CAD build for the part. Positions are in the model's coordinates, mm. A direction names the side the tool comes from. Give positions to 0.01 mm unless a question says otherwise; leave off trailing zeros. Loops run counter-clockwise (first coordinate to the right, second up) from the corner with the lowest first, then second, coordinate; pieces in that order, holes last.
Autodesk Inventor part; units mm, degrees
ref_plane "YZ Plane" through (0, 0, 0) normal (1, 0, 0) x (0, 1, 0)
ref_plane "XZ Plane" through (0, 0, 0) normal (0, 1, 0) x (-1, 0, 0)
ref_plane "XY Plane" through (0, 0, 0) normal (0, 0, 1) x (1, 0, 0)
sketch "草圖17" plane through (0, 0, 0) normal (0, 0, 1) x (1, 0, 0)
  line L0 (-12.5, -3) -> (12.5, -3)
  line L1 (12.5, -3) -> (12.5, 3)
  line L2 (12.5, 3) -> (-12.5, 3)
  line L3 (-12.5, 3) -> (-12.5, -3)
  line L4 (-12.5, -3) -> (12.5, 3) construction
  line L5 (12.5, -3) -> (-12.5, 3) construction
  line L6 (0, 0) -> (-6.6625, 0) construction
  circle A0 centre (9.5, 0) radius 2
  line L7 (-2.5, 0) -> (-4.5, 0) construction
  line L8 (-2.5, 1) -> (-4.5, 1)
  line L9 (-4.5, -1) -> (-2.5, -1)
  arc A1 (-2.5, -1) -> (-2.5, 1) centre (-2.5, 0) ccw
  arc A2 (-4.5, 1) -> (-4.5, -1) centre (-4.5, 0) ccw
  line L10 (5.5, -0.0384) -> (3.5, -0.0384) construction
  line L11 (5.5, 0.9616) -> (3.5, 0.9616)
  line L12 (3.5, -1.0384) -> (5.5, -1.0384)
  arc A3 (5.5, -1.0384) -> (5.5, 0.9616) centre (5.5, -0.0384) ccw
  arc A4 (3.5, 0.9616) -> (3.5, -1.0384) centre (3.5, -0.0384) ccw
  line L13 (7.5, 3) -> (7.5, -3)
  point P0 (-3.5, 0)
  point P1 (4.5, -0.0384)
  dimension "d166" = 25
  dimension "d167" = 6
  dimension "d170" = 4
  dimension "d171" = 3
  dimension "d173" = 2
  dimension "d174" = 12
  dimension "d175" = 2
  dimension "d190" = 4
  dimension "d191" = 2
  dimension "d192" = 2
extrude "擠出18" add sketch "草圖17" along normal mid plane 4 contours L3 L2 L13 L0
sketch "草圖18" plane through (0, 0, 0) normal (0, 0, 1) x (1, 0, 0)
  line L0 (7.5, -3) -> (-12.5, -3)
  line L1 (-12.5, -3) -> (-12.5, 3)
  line L2 (-12.5, 3) -> (7.5, 3)
  arc A0 (-2.5, -1) -> (-2.5, 1) centre (-2.5, 0) ccw
  line L3 (-2.5, 1) -> (-4.5, 1)
  arc A1 (-4.5, 1) -> (-4.5, -1) centre (-4.5, 0) ccw
  line L4 (-4.5, -1) -> (-2.5, -1)
  line L5 (-12.5, -5.1) -> (-21.5, -5.1)
  line L6 (-21.5, -5.1) -> (-21.5, 5.1)
  line L7 (-21.5, 5.1) -> (-12.5, 5.1)
  line L8 (-12.5, 5.1) -> (-12.5, -5.1)
  line L9 (-12.5, -5.1) -> (-21.5, 5.1) construction
  line L10 (-21.5, -5.1) -> (-12.5, 5.1) construction
  arc A2 (-2.5, -1) -> (-2.5, 1) centre (-2.5, 0) ccw construction
  line L11 (-2.5, 0) -> (-4.5, 0) construction
  line L12 (-21.5, 0) -> (-31.5, 0) construction
  line L13 (-21.5, 2.1) -> (-31.5, 2.1)
  line L14 (-31.5, -2.1) -> (-21.5, -2.1)
  arc A3 (-21.5, -2.1) -> (-21.5, 2.1) centre (-21.5, 0) ccw
  arc A4 (-31.5, 2.1) -> (-31.5, -2.1) centre (-31.5, 0) ccw
  line L15 (-31.5, 5.1) -> (-21.5, 5.1)
  arc A5 (-21.5, -5.1) -> (-21.5, 5.1) centre (-21.5, 0) ccw
  line L16 (-21.5, -5.1) -> (-31.5, -5.1)
  arc A6 (-31.5, 5.1) -> (-31.5, -5.1) centre (-31.5, 0) ccw
  line L17 (-12.5, -3) -> (-12.5, 3) construction
  line L18 (7.5, 3) -> (7.5, -3)
  point P0 (0, 0)
  point P1 (-17, 0)
  point P2 (-26.5, 0)
  dimension "d181" = 2.1
  dimension "d182" = 10
  dimension "d183" = 3
  dimension "d189" = 9
extrude "擠出19" add sketch "草圖18" along normal mid plane 11 contours L8 L5 A5 L7 L1 | L16 A6 L15 L6 L13 A4 L14 | L6 A3 A5
sketch "草圖19" plane through (0, 0, 0) normal (0, 0, 1) x (1, 0, 0)
  arc A0 (-31.5, 5.1) -> (-31.5, -5.1) centre (-31.5, 0) ccw
  line L0 (-31.5, 5.1) -> (-12.5, 5.1)
  line L1 (-12.5, 5.1) -> (-12.5, -5.1)
  line L2 (-12.5, -5.1) -> (-31.5, -5.1)
  arc A1 (-21.5, -2.1) -> (-21.5, 2.1) centre (-21.5, 0) ccw
  line L3 (-21.5, 2.1) -> (-31.5, 2.1)
  arc A2 (-31.5, 2.1) -> (-31.5, -2.1) centre (-31.5, 0) ccw
  line L4 (-31.5, -2.1) -> (-21.5, -2.1)
  line L5 (-15.5, -5.1) -> (-45.605, -5.1)
  line L6 (-45.605, -5.1) -> (-45.605, 5.1)
  line L7 (-45.605, 5.1) -> (-15.5, 5.1)
  line L8 (-15.5, 5.1) -> (-15.5, -5.1)
  line L9 (-31.5, 5.1) -> (-12.5, 5.1)
  point P0 (0, 0)
  point P1 (-15.5, 5.1)
  dimension "d186" = 3
extrude "擠出20" cut sketch "草圖19" along normal mid plane 7 contours L0 L8 L2 A0 | A0 L5 L6 L7
sketch "草圖20" plane through (7.5, 3, 2) normal (0, 1, 0) x (1, 0, 0)
  line L0 (0, 0) -> (-20, 0)
  line L1 (-20, 0) -> (0, 0)
  line L2 (0, 4) -> (0, 0)
  point P0 (-7.5, 2)
  dimension "d193" = 20
  dimension "d194" = 0
extrude "擠出21" [suppressed]
properties part number "fan_holder_0301"
1. Saw through at B-B, the plane x = -17. List the corners of the cut face in (y, z).
Responses:
outline: (-5.1, -5.5) - (5.1, -5.5) - (5.1, -3.5) - (-5.1, -3.5) - close; (-5.1, 3.5) - (5.1, 3.5) - (5.1, 5.5) - (-5.1, 5.5) - close
2. Saw through at C-C, the plane x = -27. List the corners of the cut face in (y, z).
Responses:
outline: (-5.1, -5.5) - (-2.1, -5.5) - (-2.1, -3.5) - (-5.1, -3.5) - close; (-5.1, 3.5) - (-2.1, 3.5) - (-2.1, 5.5) - (-5.1, 5.5) - close; (2.1, -5.5) - (5.1, -5.5) - (5.1, -3.5) - (2.1, -3.5) - close; (2.1, 3.5) - (5.1, 3.5) - (5.1, 5.5) - (2.1, 5.5) - close
3. Tool access for faces 1 (the face through (-2.6, 1.4, -2)), 2 (the face through (-3, -3, 0)), 3 (the face through (2.5, -0.1, 0)), 4 (the face through (-26.2, 2.3, -3.5)): list every direction of +Z, -Z, +X, -X, +Y, -Y with a clear straight run to the whole face (end or side of a thin tool).
Responses:
face 1: -Z, +X, +Y, -Y
face 2: +Z, -Z, +X, -Y
face 3: +Z, -Z
face 4: -X, +Y, -Y
4. Saw through at A-A, the plane z = 1.5. List the corners of the cut face in (x, y).
Responses:
outline: (-15.5, -5.1) - (-12.5, -5.1) - (-12.5, -3) - (7.5, -3) - (7.5, 3) - (-12.5, 3) - (-12.5, 5.1) - (-15.5, 5.1) - close; hole (-4.5, -1) - (-2.5, -1) arc R1 ccw to (-2.5, 1) - (-4.5, 1) arc R1 ccw to start; hole (3.5, -1.04) - (5.5, -1.04) arc R1 ccw to (5.5, 0.96) - (3.5, 0.96) arc R1 ccw to start
5. Saw through at D-D, the plane z = 4.5. List the corners of the cut face in (x, y), and give its area (3 significant figures).
Responses:
outline: (-31.5, -5.1) - (-12.5, -5.1) - (-12.5, 5.1) - (-31.5, 5.1) arc R5.1 ccw to start; hole (-31.5, -2.1) - (-21.5, -2.1) arc R2.1 ccw to (-21.5, 2.1) - (-31.5, 2.1) arc R2.1 ccw to start
area: 179 mm2
6. Probe line 1 along Z through (x, y) = (-23, 4.5); line 2 along Y through (x, z) = (-29.5, 5.25); line 3 along X through (y, z) = (0, 5.25). List the from-to ranges inside material, lowest first.
Responses:
line 1: z = -5.5 to -3.5, 3.5 to 5.5
line 2: y = -5.1 to -2.1, 2.1 to 5.1
line 3: x = -36.6 to -33.6, -19.4 to -12.5
7. Pull direction Z, two halves, no side cores. Call faces 5 (the face through (-15.5, 0, 0)), 6 (the face through (-24.7, 2.3, 5.5)), 7 (the face through (-1.5, 0, 0)): released by +Z, released by -Z, zero draft, split by the parting line, or undercut.
Responses:
face 5: undercut
face 6: released by +Z
face 7: zero draft
8. Drop flat-ended pins along their axis: pin 1 (4.5 mm diameter, centred on x = -7, z = 0.5, fed in from +Y); pin 2 (3 mm diameter, centred on x = -4, y = 0, fed in from -Z); pin 3 (3 mm diameter, centred on x = -5.5, z = 0, fed in from -Y); pin 4 (3 mm diameter, centred on x = -25, z = 1.5, fed in from -Y). Give the stop position or say it passes through.
Responses:
pin 1: stops at y = 3
pin 2: stops at z = -2
pin 3: stops at y = -3
pin 4: passes through
